from build123d import *

# Parameters (mm, degrees)
F1_DEPTH = 6.35
F3_DEPTH = 7.112
F5_DEPTH = 7.62
F6_DEPTH = 8.128


with BuildPart() as f1:
    # F0 (on Front) → F1 (new body)
    with BuildSketch(Plane.XZ):
        with BuildLine():
            ThreePointArc((1.7938007368, 13.1640341133), (0, 13.6572233107), (-1.7938007368, 13.1640341133))
            ThreePointArc((-1.7938007368, 13.1640341133), (-5.3164680529, 19.2534781495), (-12.3440632597, 19.5750668645))
            ThreePointArc((-12.3440632597, 19.5750668645), (-16.2697935097, 14.9604002099), (-16.5348500013, 8.9076114818))
            ThreePointArc((-16.5348500013, 8.9076114818), (-20.8041441001, 5.2034101528), (-23.0115186423, 0))
            ThreePointArc((-23.0115186423, 0), (-21.7531756781, -5.1696394341), (-18.0587712675, -8.9984741062))
            ThreePointArc((-18.0587712675, -8.9984741062), (-13.693909696, -11.7987149183), (-8.8199935853, -13.5702416301))
            ThreePointArc((-8.8199935853, -13.5702416301), (-4.4612425903, -14.5759230892), (0, -14.9036729708))
            ThreePointArc((0, -14.9036729708), (4.4612425903, -14.5759230892), (8.8199935853, -13.5702416301))
            ThreePointArc((8.8199935853, -13.5702416301), (13.693909696, -11.7987149183), (18.0587712675, -8.9984741062))
            ThreePointArc((18.0587712675, -8.9984741062), (21.7531756781, -5.1696394341), (23.0115186423, 0))
            ThreePointArc((23.0115186423, 0), (20.8041441001, 5.2034101528), (16.5348500013, 8.9076114818))
            ThreePointArc((16.5348500013, 8.9076114818), (16.2697935097, 14.9604002099), (12.3440632597, 19.5750668645))
            ThreePointArc((12.3440632597, 19.5750668645), (5.3164680529, 19.2534781495), (1.7938007368, 13.1640341133))
        make_face()
    extrude(amount=F1_DEPTH)

    # F2 (on Front) → F3 (join)
    with BuildSketch(Plane.XZ):
        with BuildLine():
            add(Edge.make_bspline(
                [(-9.6370028332, 18.2963684201), (-17.5014538427, 18.2963684201), (-13.569228338, 8.9325434528), (-9.6370028332, -0.4312815145), (-5.7047773284, 8.9325434528), (-1.7725518236, 18.2963684201), (-9.6370028332, 18.2963684201)],
                knots=[0, 0, 0, 2.0943951024, 2.0943951024, 4.1887902048, 4.1887902048, 6.2831853072, 6.2831853072, 6.2831853072], degree=2, weights=[1, 0.5, 1, 0.5, 1, 0.5, 1]))
        make_face()
        with BuildLine():
            add(Edge.make_bspline(
                [(-2.4665053934, 0.8340993081), (-3.5359200187, 0.8340993081), (-3.001212706, -0.4170496541), (-2.4665053934, -1.6681986162), (-1.9317980807, -0.4170496541), (-1.3970907681, 0.8340993081), (-2.4665053934, 0.8340993081)],
                knots=[0, 0, 0, 2.0943951024, 2.0943951024, 4.1887902048, 4.1887902048, 6.2831853072, 6.2831853072, 6.2831853072], degree=2, weights=[1, 0.5, 1, 0.5, 1, 0.5, 1]))
        make_face()
        with BuildLine():
            add(Edge.make_bspline(
                [(9.6370028332, 18.2963684201), (1.7725518236, 18.2963684201), (5.7047773284, 8.9325434528), (9.6370028332, -0.4312815145), (13.569228338, 8.9325434528), (17.5014538427, 18.2963684201), (9.6370028332, 18.2963684201)],
                knots=[0, 0, 0, 2.0943951024, 2.0943951024, 4.1887902048, 4.1887902048, 6.2831853072, 6.2831853072, 6.2831853072], degree=2, weights=[1, 0.5, 1, 0.5, 1, 0.5, 1]))
        make_face()
        with BuildLine():
            add(Edge.make_bspline(
                [(2.4665053934, 0.8340993081), (1.3970907681, 0.8340993081), (1.9317980807, -0.4170496541), (2.4665053934, -1.6681986162), (3.001212706, -0.4170496541), (3.5359200187, 0.8340993081), (2.4665053934, 0.8340993081)],
                knots=[0, 0, 0, 2.0943951024, 2.0943951024, 4.1887902048, 4.1887902048, 6.2831853072, 6.2831853072, 6.2831853072], degree=2, weights=[1, 0.5, 1, 0.5, 1, 0.5, 1]))
        make_face()
        with BuildLine():
            ThreePointArc((0, -7.315651048), (-6.1209625513, -6.4094895832), (-11.7790261284, -3.9047684986))
            ThreePointArc((-11.7790261284, -3.9047684986), (-6.8239147975, -8.7429084856), (0, -9.9239731207))
            ThreePointArc((0, -9.9239731207), (6.8239147975, -8.7429084856), (11.7790261284, -3.9047684986))
            ThreePointArc((11.7790261284, -3.9047684986), (6.1209625513, -6.4094895832), (0, -7.315651048))
        make_face()
    extrude(amount=F3_DEPTH)

    # F4 (on Front) → F5 (join)
    with BuildSketch(Plane.XZ):
        with BuildLine():
            add(Edge.make_bspline(
                [(-9.7133507952, 16.7924873531), (-15.5296298908, 16.7924873531), (-12.621490343, 9.5717669465), (-9.7133507952, 2.3510465398), (-6.8052112474, 9.5717669465), (-3.8970716996, 16.7924873531), (-9.7133507952, 16.7924873531)],
                knots=[0, 0, 0, 2.0943951024, 2.0943951024, 4.1887902048, 4.1887902048, 6.2831853072, 6.2831853072, 6.2831853072], degree=2, weights=[1, 0.5, 1, 0.5, 1, 0.5, 1]))
        make_face()
        with BuildLine():
            add(Edge.make_bspline(
                [(9.7133507952, 16.7924873531), (3.8970716996, 16.7924873531), (6.8052112474, 9.5717669465), (9.7133507952, 2.3510465398), (12.621490343, 9.5717669465), (15.5296298908, 16.7924873531), (9.7133507952, 16.7924873531)],
                knots=[0, 0, 0, 2.0943951024, 2.0943951024, 4.1887902048, 4.1887902048, 6.2831853072, 6.2831853072, 6.2831853072], degree=2, weights=[1, 0.5, 1, 0.5, 1, 0.5, 1]))
        make_face()
    extrude(amount=F5_DEPTH)

    # F4 (on Front) → F6 (join)
    with BuildSketch(Plane.XZ):
        with BuildLine():
            add(Edge.make_bspline(
                [(-9.7133507952, 16.7924873531), (-15.5296298908, 16.7924873531), (-12.621490343, 9.5717669465), (-9.7133507952, 2.3510465398), (-6.8052112474, 9.5717669465), (-3.8970716996, 16.7924873531), (-9.7133507952, 16.7924873531)],
                knots=[0, 0, 0, 2.0943951024, 2.0943951024, 4.1887902048, 4.1887902048, 6.2831853072, 6.2831853072, 6.2831853072], degree=2, weights=[1, 0.5, 1, 0.5, 1, 0.5, 1]))
        make_face()
        with BuildLine():
            add(Edge.make_bspline(
                [(9.7133507952, 16.7924873531), (3.8970716996, 16.7924873531), (6.8052112474, 9.5717669465), (9.7133507952, 2.3510465398), (12.621490343, 9.5717669465), (15.5296298908, 16.7924873531), (9.7133507952, 16.7924873531)],
                knots=[0, 0, 0, 2.0943951024, 2.0943951024, 4.1887902048, 4.1887902048, 6.2831853072, 6.2831853072, 6.2831853072], degree=2, weights=[1, 0.5, 1, 0.5, 1, 0.5, 1]))
        make_face()
    extrude(amount=F6_DEPTH)


solid = f1.part
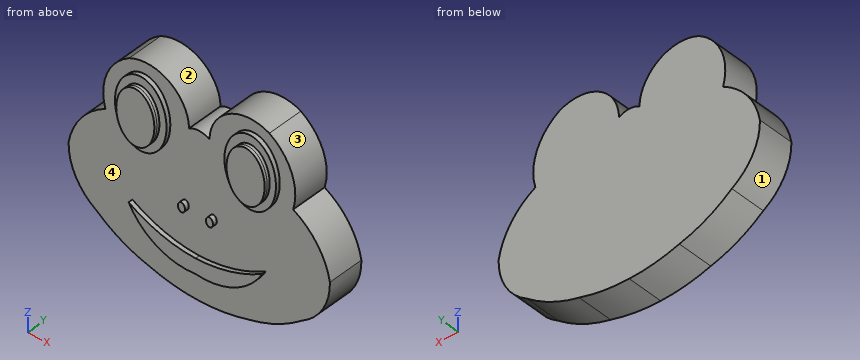
The model under review builds one solid part; all positions refer to its coordinate system, in mm. Face numbers are marked on the shaded views. Give positions to 0.01 mm unless a question says otherwise; leave off trailing zeros. Order: outer loops, then holes, each group sorted by start corner. A loop starts at its lowest first (then second) coordinate and runs counter-clockwise, first axis right, second up. Notation, with made-up numbers: M -28,15 L 29,15 A25 cw 29,32 Z; hole C 89.25,-4 d7. An arc over 180 degrees is marked long. Answer in a Markdown table with one row per item. Add a question column.
1. Add section B-B on y = -5.5. State the section outline as (x, z) points.
2. To check wall thickness, follow line 1 along Y through (x, z) = (15.5, -8.5); line 2 along X through (y, z) = (-7.25, 10); line 3 along Y through (x, z) = (9, -5.5). State the ranges of each line that lie inside material, in increasing order.
3. For pin 1 Ø0.6 at (x, z) = (2.5, 0) entering from -Y; pin 2 Ø3 at (x, z) = (4.5, 1.5) entering from -Y; pin 3 Ø3 at (x, y) = (3.5, -5.5) entering from -Z, all flat-tipped, find the tip position at first contact; note any pin that passes through.
4. Add section C-C on x = 16. State the section outline as (y, z) points, plus the area to 3 significant figures.
5. Add section D-D on x = -19. State the section outline as (y, z) points.
6. Mouldability with a two-part tool opening along X and no side actions: class the marked faces 1, 2, 3 and 4 as released by +X, released by -X, zero draft, split by the parting line, or undercut.
7. Add section A-A on z = -8. State the section outline as (x, y) points.
The answers:
| question | item | result |
|---|---|---|
| 1 | outline | M -23.01,0 A10.18 ccw -18.06,-9 A23.43 ccw -8.82,-13.57 A29.18 ccw 0,-14.9 A29.18 ccw 8.82,-13.57 A23.43 ccw 18.06,-9 A10.18 ccw 23.01,0 A12.53 ccw 16.53,8.91 A9.33 ccw 12.34,19.58 A7.33 ccw 1.79,13.16 A3.51 ccw -1.79,13.16 A7.33 ccw -12.34,19.58 A9.33 ccw -16.53,8.91 A12.53 ccw Z |
| 2 | line 1 | -6.35 to 0 |
| 2 | line 2 | -12.77 to -6.65, 6.65 to 12.77 |
| 2 | line 3 | -7.11 to 0 |
| 3 | pin 1 | y = -7.11 |
| 3 | pin 2 | y = -6.35 |
| 3 | pin 3 | z = -14.84 |
| 4 | outline | M -6.35,-10.49 L 0,-10.49 L 0,15.58 L -6.35,15.58 Z |
| 4 | area | 166 mm2 |
| 5 | outline | M -6.35,-8.36 L 0,-8.36 L 0,7.19 L -6.35,7.19 Z |
| 6 | face 1 | released by -X |
| 6 | face 2 | undercut |
| 6 | face 3 | released by +X |
| 6 | face 4 | undercut |
| 7 | outline | M -19.45,-6.35 L -8.08,-6.35 L -8.08,-7.11 L 8.08,-7.11 L 8.08,-6.35 L 19.45,-6.35 L 19.45,0 L -19.45,0 Z |
